The drawing under review shows one solid part. Ordinate dimensions are in mm from its lowest x, y, z. Coordinates: 2 decimals unless noted, no trailing zeros. Order: outer loops, then holes, each group sorted by start corner. A loop starts at its lowest first (then second) coordinate and runs counter-clockwise, first axis right, second up. Notation, with made-up numbers: (-36, 5.5) -> (-12, 5.5) arc R19 ccw to (-12, 34.5) -> close; hole circle Ø3 at (74, 32). An arc over 180 degrees is marked (long way). Use a Markdown table: item, result. Add a question column.
Q1. Add section A-A (y = 4). State the section outline as (x, z) points (1 decimal).
Q2. The part is to be moulded in two halves that separate along X. For the marked faces 1, 2 and 3, say which applies: pulls with the +X half, pulls with the -X half, needs draft (parallel to the pull), parting line crosses it, or undercut.
Q3. Add section C-C (z = 4). State the section outline as (x, y) points (1 decimal).
Q4. Add section D-D (y = 0.5). State the section outline as (x, z) points.
Q5. Add section B-B (x = 47). State the section outline as (y, z) points.
Q6. Wall thickness on probe 1 along Y at (x, z) = (47, 2.2); probe 2 along Z at (x, y) = (48, 6); probe 3 along X at (y, z) = (6.75, 4.5): over which ranges is each line inside the solid? List them lowest first.
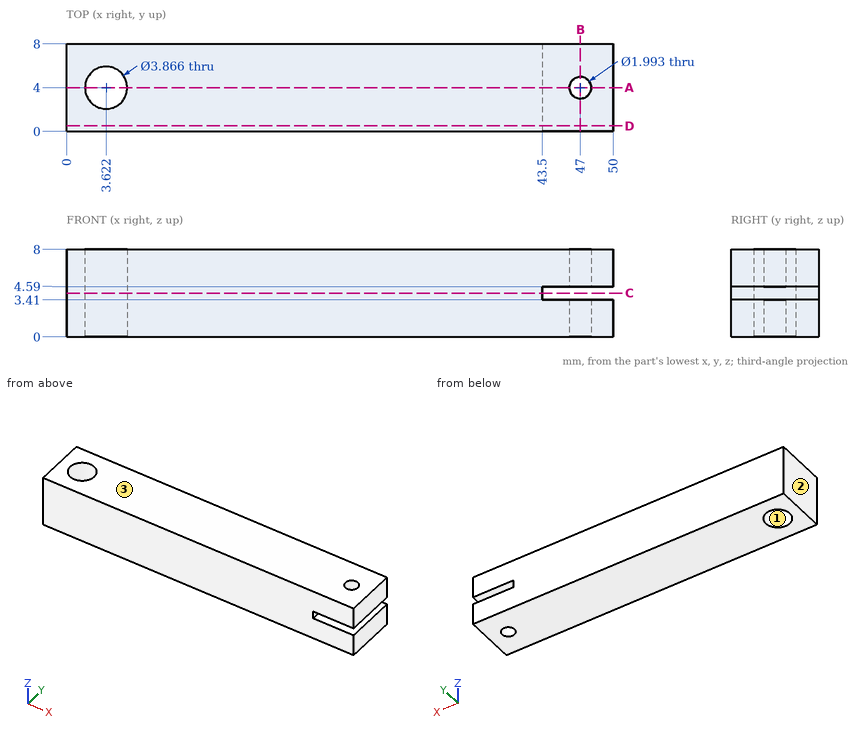
Established:
| question | item | result |
|---|---|---|
| 1 | outline | (0, 0) -> (1.7, 0) -> (1.7, 8) -> (0, 8) -> close; (5.6, 0) -> (46, 0) -> (46, 3.4) -> (43.5, 3.4) -> (43.5, 4.6) -> (46, 4.6) -> (46, 8) -> (5.6, 8) -> close; (48, 0) -> (50, 0) -> (50, 3.4) -> (48, 3.4) -> close; (48, 4.6) -> (50, 4.6) -> (50, 8) -> (48, 8) -> close |
| 2 | face 1 | undercut |
| 2 | face 2 | pulls with the -X half |
| 2 | face 3 | needs draft |
| 3 | outline | (0, 0) -> (43.5, 0) -> (43.5, 8) -> (0, 8) -> close; hole circle Ø3.9 at (3.6, 4) |
| 4 | outline | (0, 0) -> (50, 0) -> (50, 3.41) -> (43.5, 3.41) -> (43.5, 4.59) -> (50, 4.59) -> (50, 8) -> (0, 8) -> close |
| 5 | outline | (0, 0) -> (3, 0) -> (3, 3.41) -> (0, 3.41) -> close; (0, 4.59) -> (3, 4.59) -> (3, 8) -> (0, 8) -> close; (5, 0) -> (8, 0) -> (8, 3.41) -> (5, 3.41) -> close; (5, 4.59) -> (8, 4.59) -> (8, 8) -> (5, 8) -> close |
| 6 | probe 1 | 0 to 3, 5 to 8 |
| 6 | probe 2 | 0 to 3.41, 4.59 to 8 |
| 6 | probe 3 | 0 to 43.5 |
